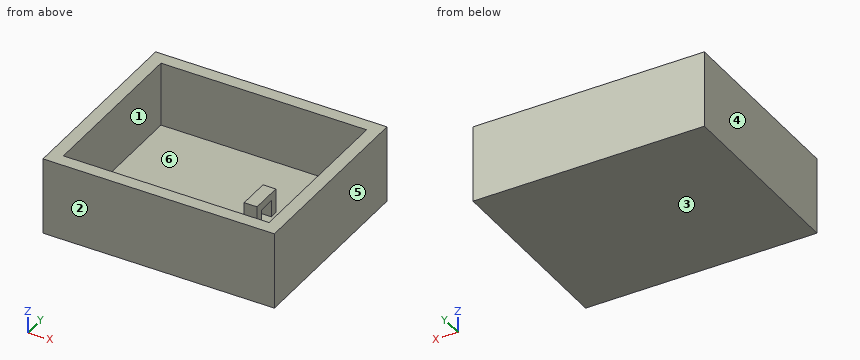
Autodesk Inventor part; units mm, degrees
ref_plane "YZ Plane" through (0, 0, 0) normal (1, 0, 0) x (0, 1, 0)
ref_plane "XZ Plane" through (0, 0, 0) normal (0, 1, 0) x (-1, 0, 0)
ref_plane "XY Plane" through (0, 0, 0) normal (0, 0, 1) x (1, 0, 0)
sketch "Skizze1" plane through (0, 0, 0) normal (0, 0, 1) x (1, 0, 0)
  line L0 (-18, 0) -> (108, 0)
  line L1 (0, -15) -> (0, 90)
  line L2 (0, 0) -> (90, 0)
  line L3 (90, 0) -> (90, 75)
  line L4 (90, 75) -> (0, 75)
  line L5 (0, 75) -> (0, 0)
  line L6 (5, 70) -> (85, 70)
  line L7 (85, 70) -> (85, 5)
  line L8 (85, 5) -> (5, 5)
  line L9 (5, 5) -> (5, 70)
  point P0 (0, 75)
  dimension "d0" = 75
  dimension "d1" = 90
  dimension "d2" = 5
  dimension "d3" = 5
  dimension "d4" = 5
  dimension "d5" = 5
extrude "Extrusion1" add sketch "Skizze1" along normal blind 25
sketch "Skizze2" plane through (0, 0, 0) normal (0, 0, -1) x (-1, 0, 0)
  line L0 (0, 75) -> (0, 0)
  line L1 (0, 75) -> (-90, 75)
  line L2 (-90, 75) -> (-90, 0)
  line L3 (-90, 0) -> (0, 0)
  line L4 (0, 0) -> (0, 75)
extrude "Extrusion2" add sketch "Skizze2" along normal blind 5
sketch "Skizze3" plane through (0, 0, 0) normal (0, 0, 1) x (1, 0, 0)
  line L0 (60, 31.25) -> (65, 31.25)
  line L1 (65, 31.25) -> (65, 43.75)
  line L2 (65, 43.75) -> (60, 43.75)
  line L3 (60, 43.75) -> (60, 31.25)
  line L4 (85, 5) -> (5, 5)
  line L5 (5, 5) -> (5, 70)
  point P0 (0, 0)
  dimension "d10" = 12.5
  dimension "d11" = 5
  dimension "d12" = 26.25
  dimension "d13" = 55
extrude "Extrusion3" add sketch "Skizze3" along normal blind 9.5
sketch "Skizze4" plane through (60, 31.25, 0) normal (-1, 0, 0) x (0, 0, 1)
  line L0 (0, 12.5) -> (0, 0)
  line L1 (0, 3) -> (6.5, 3)
  line L2 (6.5, 3) -> (6.5, 9.5)
  line L3 (6.5, 9.5) -> (0, 9.5)
  line L4 (0, 9.5) -> (0, 3)
  line L5 (0, 0) -> (9.5, 0)
  point P0 (0, -31.25)
  point P1 (0, 9.5)
  dimension "d16" = 6.5
  dimension "d17" = 6.5
  dimension "d18" = 3
extrude "Extrusion4" cut sketch "Skizze4" against normal blind 5
properties part number "Wasserbecken" material "Acetalharz, Schwarz"
The listing builds one solid part. Answer for the finished solid, in the listing's coordinates (mm). Face numbers are marked on the shaded views. A direction names the side the tool comes from. Coordinates: 2 decimals unless noted, no trailing zeros. Write each loop counter-clockwise with the first axis right and the second up, starting at its lowest first coordinate (ties: lowest second). Pieces come first, ordered by that corner, then holes. Notation, with made-up numbers: (9.5, -39.5) - (60.5, -39.5) arc R25 ccw to (60.5, -10.5) - close; hole circle Ø7 at (-36.75, 83.25). An arc over 180 degrees is marked (long way). Return JSON: item names as keys, results as strings. Group by question number.
1. A cutting plane is placed at B-B, the plane x = 62. Determine the outline of the cut face in (y, z).
2. Which of the six approach directions +Z, -Z, +X, -X, +Y, -Y give full straight-line access (tool end or side, diameter ignored) to the marked faces 1 and 2?
3. Determine the mould class of the marked faces 3, 4, 5 and 6 for opening direction X: released by +X, released by -X, zero draft, split by the parting line, or undercut.
4. A cutting plane is placed at D-D, the plane x = 44. Determine the outline of the cut face in (y, z).
5. A cutting plane is placed at C-C, the plane y = 13.5. Determine the outline of the cut face in (x, z), plus the area to 3 significant figures.
6. Straight lines are drawn through the part: L1, parallel to X at y = 42, z = 3.75; L2, parallel to Y at x = 59.5, z = 5.75; L3, parallel to X at y = 48.5, z = 22.25. For each, find the intervals that lie inside material, in ascending order.
7. A cutting plane is placed at A-A, the plane z = 7.75. Determine the outline of the cut face in (x, y), plus the area to 3 significant figures.
8. Given pin 1 (4 mm diameter, centred on x = 61.5, y = 38, fed in from +Z); pin 2 (1.5 mm diameter, centred on x = 17.5, y = 37.5, fed in from +Z), each flat-ended and moving along its own axis, determine where each tip first touches the part or whether it passes through.
Ans:
{
 "1": {"outline": "(0, -5) - (75, -5) - (75, 25) - (70, 25) - (70, 0) - (43.75, 0) - (43.75, 9.5) - (31.25, 9.5) - (31.25, 0) - (5, 0) - (5, 25) - (0, 25) - close; hole (34.25, 0) - (40.75, 0) - (40.75, 6.5) - (34.25, 6.5) - close"},
 "2": {"face 1": "+Z", "face 2": "+Z, -Z, +X, -X, -Y"},
 "3": {"face 3": "zero draft", "face 4": "released by -X", "face 5": "released by +X", "face 6": "undercut"},
 "4": {"outline": "(0, -5) - (75, -5) - (75, 25) - (70, 25) - (70, 0) - (5, 0) - (5, 25) - (0, 25) - close"},
 "5": {"outline": "(0, -5) - (90, -5) - (90, 25) - (85, 25) - (85, 0) - (5, 0) - (5, 25) - (0, 25) - close", "area": "700 mm²"},
 "6": {"L1": "0 to 5, 60 to 65, 85 to 90", "L2": "0 to 5, 70 to 75", "L3": "0 to 5, 85 to 90"},
 "7": {"outline": "(0, 0) - (90, 0) - (90, 75) - (0, 75) - close; (60, 31.25) - (65, 31.25) - (65, 43.75) - (60, 43.75) - close; hole (5, 5) - (85, 5) - (85, 70) - (5, 70) - close", "area": "1,610 mm²"},
 "8": {"pin 1": "z = 9.5", "pin 2": "z = 0"}
}
